Check sheet for the modelled part. Datum: model origin and axes. Units: mm. A direction names the side the tool comes from. Round coordinates to 2 decimals unless told otherwise and drop trailing zeros. Order: outer loops, then holes, each group sorted by start corner. A loop starts at its lowest first (then second) coordinate and runs counter-clockwise, first axis right, second up.
Q1. Set-up check for faces 4 (the flat face through (-10, -1, -9.675)), 5 (the flat face through (10, -3, 12)), 6 (the conical face through (-23.43, -1.19, -36.24)): record each of +Z, -Z, +X, -X, +Y, -Y from which the full face is reachable in a straight line by a thin tool's end or side.
Q2. Cross-section at C-C on x = 12.6. Record the cut outline in (y, z) (3 decimals).
Q3. Cross-section at B-B on x = 6.5. Record the cut outline in (y, z) (3 decimals), then the cut area to 3 significant figures.
Q4. Scan lines: probe 1 along Z at (x, y) = (12.6, -3.4) (3 decimals); probe 2 along X at (y, z) = (-3.35, -24.45); probe 3 along Z at (x, y) = (15, -0.2) (3 decimals). Record each from-to range of solid material in increasing order.
Q5. Cross-section at D-D on z = -24.45. Record the cut outline in (x, y), then the cut area to 3 significant figures.
Q6. Mould release check, pull along Z, two halves, no side actions. Record for faces 1 (the flat face through (0.272, -1.521, -38.196)), 2 (the flat face through (0, 0, -10)), 3 (the flat face through (-3.55, -2, 0)): +Z half, -Z half, draft (parallel to the pull), parting line (faces both ways), or undercut.
Q7. Depth check by flat-ended pin: P1, Ø2, axis at y = -1.5, z = 1.5, coming from the +X side; P2, Ø9.5, axis at x = -4.5, z = -20.5, coming from the +Y side; P3, Ø2, axis at x = -9, y = -1.5, coming from the -Z side (3 decimals). Enter the tip coordinate at first touch or a pass-through.
Q8. Cross-section at A-A on z = 7.5. Record the cut outline in (x, y), then the cut area to 3 significant figures.
from build123d import *

# Parameters (mm, degrees)
SKETCH1_W                                     = 53.9
SKETCH1_H                                     = 59.675
SKETCH1_W_2                                   = 12.9
SKETCH1_H_2                                   = 19.35
BOSS_EXTRUDE1_DEPTH                           = 4
FILLET1_R                                     = 7.5
CHAMFER1_SIZE                                 = 3
CUT_EXTRUDE1_START                            = -2
SKETCH4_W                                     = 12.9
SKETCH4_H                                     = 24
CUT_EXTRUDE1_DEPTH                            = 3
SKETCH5_W                                     = 41.2
SKETCH5_H                                     = 18.9
CUT_EXTRUDE2_DEPTH                            = 0.25
CSK_FOR_8_FLAT_HEAD_SOCKET_CAP_SCREW1_A_COUNT = 2
CSK_FOR_8_FLAT_HEAD_SOCKET_CAP_SCREW1_A_PITCH = 25.2


with BuildPart() as part:
    # Sketch1 → Boss-Extrude1 (new body)
    with BuildSketch(Plane(origin=(0, 0, 0), x_dir=(1, 0, 0), z_dir=(0, 1, 0))):
        with Locations((0, 9.8375)):
            Rectangle(SKETCH1_W, SKETCH1_H)
        with Locations((10, 0)):
            Rectangle(SKETCH1_W_2, SKETCH1_H_2, mode=Mode.SUBTRACT)
        with Locations((-10, 0)):
            Rectangle(SKETCH1_W_2, SKETCH1_H_2, mode=Mode.SUBTRACT)
    extrude(amount=-BOSS_EXTRUDE1_DEPTH)

    # Fillet1
    fillet1_edges = [part.edges().sort_by_distance(p)[0] for p in [
        (26.95, -2, 20),
        (-26.95, -2, 20),
        (-26.95, -2, -39.675),
        (26.95, -2, -39.675),
    ]]
    fillet(fillet1_edges, radius=FILLET1_R)

    # Chamfer1
    chamfer1_edges = [part.edges().sort_by_distance(p)[0] for p in [
        (26.95, 0, -9.8375),
        (0, 0, -39.675),
        (-26.95, 0, -9.8375),
        (0, 0, 20),
        (-24.753300859, 0, 17.803300859),
        (24.753300859, 0, 17.803300859),
        (-24.753300859, 0, -37.478300859),
        (24.753300859, 0, -37.478300859),
    ]]
    chamfer(chamfer1_edges, length=CHAMFER1_SIZE)

    # Sketch4 → Cut-Extrude1 (cut, through all)
    with BuildSketch(Plane(origin=(0, 0, 0), x_dir=(1, 0, 0), z_dir=(0, 1, 0)).offset(CUT_EXTRUDE1_START)):
        with Locations((-10, 0)):
            Rectangle(SKETCH4_W, SKETCH4_H)
        with Locations((10, 0)):
            Rectangle(SKETCH4_W, SKETCH4_H)
    extrude(amount=-CUT_EXTRUDE1_DEPTH, mode=Mode.SUBTRACT)

    # Sketch5 → Cut-Extrude2 (cut)
    with BuildSketch(Plane(origin=(0, 0, 0), x_dir=(1, 0, 0), z_dir=(0, 1, 0))):
        with Locations((0, 24.45)):
            Rectangle(SKETCH5_W, SKETCH5_H)
    extrude(amount=-CUT_EXTRUDE2_DEPTH, mode=Mode.SUBTRACT)

    # Sketch3 → CSK for #8 Flat Head Socket Cap Screw1 (revolve, cut)
    with BuildSketch(Plane(origin=(-12.6, -0.25, -24.45), x_dir=(0, 0, 1), z_dir=(1, 0, 0))):
        Polygon((0, 0), (0, 3.75), (2.2479, 3.75), (2.2479, 2.658961536), (4.5593, 0), align=None)
    csk_for_8_flat_head_socket_cap_screw1 = revolve(axis=Axis((-12.6, 6.1, -24.45), (0, -1, 0)), mode=Mode.SUBTRACT)

    # CSK for #8 Flat Head Socket Cap Screw1 a: CSK for #8 Flat Head Socket Cap Screw1 ×2
    with Locations(*[(i * CSK_FOR_8_FLAT_HEAD_SOCKET_CAP_SCREW1_A_PITCH, 0, 0) for i in range(1, CSK_FOR_8_FLAT_HEAD_SOCKET_CAP_SCREW1_A_COUNT)]):
        add(csk_for_8_flat_head_socket_cap_screw1, mode=Mode.SUBTRACT)


solid = part.part
Results found:
1. face 4: +Y, -Y
1. face 5: -Y
1. face 6: -Z, -X, +Y
2. outline: (-4, -39.675) - (-3, -39.675) - (0, -36.675) - (0, -33.9) - (-0.25, -33.9) - (-0.25, -29.009) - (-2.909, -26.698) - (-4, -26.698) - close; (-4, -22.202) - (-2.909, -22.202) - (-0.25, -19.891) - (-0.25, -15) - (0, -15) - (0, -9.675) - (-2, -9.675) - (-2, -12) - (-4, -12) - close; (-4, 12) - (-2, 12) - (-2, 9.675) - (0, 9.675) - (0, 17) - (-3, 20) - (-4, 20) - close
3. outline: (-4, -39.675) - (-3, -39.675) - (0, -36.675) - (0, -33.9) - (-0.25, -33.9) - (-0.25, -15) - (0, -15) - (0, -9.675) - (-2, -9.675) - (-2, -12) - (-4, -12) - close; (-4, 12) - (-2, 12) - (-2, 9.675) - (0, 9.675) - (0, 17) - (-3, 20) - (-4, 20) - close
3. area: 138 mm2
4. probe 1: z = -39.675 to -26.698, -22.202 to -12, 12 to 20
4. probe 2: x = -26.95 to -14.85, -10.35 to 10.35, 14.85 to 26.95
4. probe 3: z = -36.875 to -33.9, -15 to -9.675, 9.675 to 17.2
5. outline: (-26.95, -4) - (-14.85, -4) - (-14.85, -2.91) - (-17.16, -0.25) - (-20.6, -0.25) - (-20.6, 0) - (-23.95, 0) - (-26.95, -3) - close; (-10.35, -4) - (10.35, -4) - (10.35, -2.91) - (8.04, -0.25) - (-8.04, -0.25) - (-10.35, -2.91) - close; (14.85, -4) - (26.95, -4) - (26.95, -3) - (23.95, 0) - (20.6, 0) - (20.6, -0.25) - (17.16, -0.25) - (14.85, -2.91) - close
5. area: 150 mm2
6. face 1: -Z half
6. face 2: draft
6. face 3: undercut
7. P1: stops at x = 26.45
7. P2: stops at y = -0.25
7. P3: stops at z = -39.175
8. outline: (-26.95, -4) - (-16.45, -4) - (-16.45, 0) - (-23.95, 0) - (-26.95, -3) - close; (-3.55, -4) - (3.55, -4) - (3.55, 0) - (-3.55, 0) - close; (16.45, -4) - (26.95, -4) - (26.95, -3) - (23.95, 0) - (16.45, 0) - close
8. area: 103 mm2
